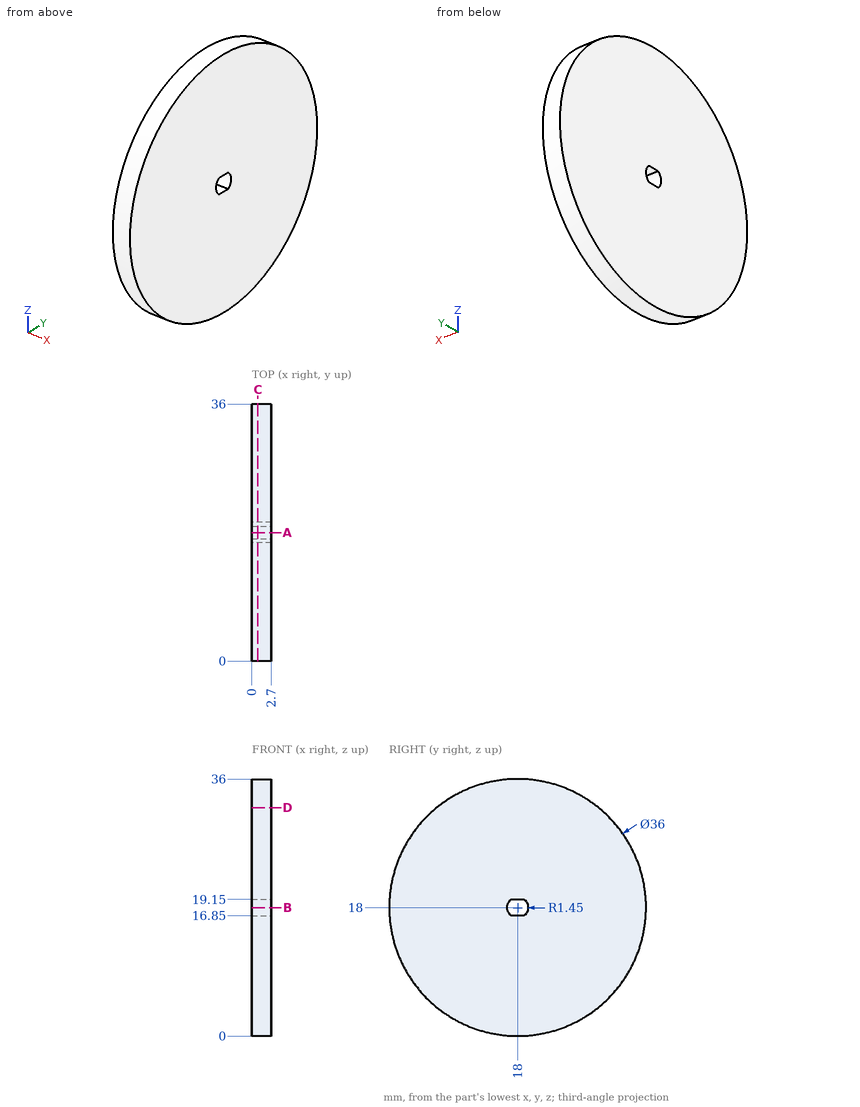
Could you check a few things on this drawing? It's one solid part, dimensions in mm from its lowest x, y, z. Round coordinates to 2 decimals unless told otherwise and drop trailing zeros. Order: outer loops, then holes, each group sorted by start corner. A loop starts at its lowest first (then second) coordinate and runs counter-clockwise, first axis right, second up. Notation, with made-up numbers: M 28.25,2.5 L 49.25,2.5 A30 cw 49.25,38.5 Z; hole C 27.25,22.25 d7. An arc over 180 degrees is marked long. Return JSON: item names as keys, results as strings. Group by question number.
1. Please list where these lines run through material, in increasing order: probe 1 along Y at (x, z) = (1.05, 17); probe 2 along Y at (x, z) = (1.2, 21.5).
2. If we section it at A-A on y = 18: List the corners of the cut face in (x, z) for me.
3. I'm going to push flat-ended pins straight in: pin 1 Ø1.5 at (x, y) = (1, 12.5) entering from +Z; pin 2 Ø1 at (x, y) = (1, 4.5) entering from -Z. Where does each tip first touch, or does it pass through?
4. If we section it at C-C on x = 0.85: List the corners of the cut face in (y, z) for me, then the cut area to 3 significant figures.
5. If we section it at B-B on z = 18: List the corners of the cut face in (x, y) for me, then the cut area to 3 significant figures.
6. If we section it at D-D on z = 32: List the corners of the cut face in (x, y) for me.
Reply:
{
 "1": {"probe 1": "0.03 to 16.95, 19.05 to 35.97", "probe 2": "0.34 to 35.66"},
 "2": {"outline": "M 0,0 L 2.7,0 L 2.7,16.85 L 0,16.85 Z; M 0,19.15 L 2.7,19.15 L 2.7,36 L 0,36 Z"},
 "3": {"pin 1": "z = 35.36", "pin 2": "z = 5.55"},
 "4": {"outline": "C 18,18 d36; hole M 17.12,16.85 L 18.88,16.85 A1.45 ccw 18.88,19.15 L 17.12,19.15 A1.45 ccw Z", "area": "1,010 mm^2"},
 "5": {"outline": "M 0,0 L 2.7,0 L 2.7,16.55 L 0,16.55 Z; M 0,19.45 L 2.7,19.45 L 2.7,36 L 0,36 Z", "area": "89.4 mm^2"},
 "6": {"outline": "M 0,6.69 L 2.7,6.69 L 2.7,29.31 L 0,29.31 Z"}
}
